Model file for the job. Use its own axes, mm. A direction names the side the tool comes from. Give positions to 0.01 mm unless a question says otherwise; leave off trailing zeros. Write each loop counter-clockwise with the first axis right and the second up, starting at its lowest first coordinate (ties: lowest second). Pieces come first, ordered by that corner, then holes. Notation, with made-up numbers: (64.25, -23.5) - (121.25, -23.5) arc R24 cw to (121.25, -12.5) - close; hole circle Ø10 at (-10, 87). An arc over 180 degrees is marked (long way). Use CSV: the item, a comma, the result in double quotes.
from build123d import *

# Parameters (mm, degrees)
SKETCH1_W           = 55
SKETCH1_H           = 46
SKETCH1_W_2         = 40
SKETCH1_H_2         = 30
BOSS_EXTRUDE1_DEPTH = 6
SKETCH3_R           = 3.556
CUT_EXTRUDE1_DEPTH  = 24
SKETCH6_W           = 12
SKETCH6_H           = 12
CUT_EXTRUDE4_DEPTH  = 4
FILLET1_R           = 10


with BuildPart() as part:
    # Sketch1 → Boss-Extrude1 (new body, symmetric)
    with BuildSketch(Plane.XY):
        Rectangle(SKETCH1_W, SKETCH1_H)
        Rectangle(SKETCH1_W_2, SKETCH1_H_2, mode=Mode.SUBTRACT)
    extrude(amount=BOSS_EXTRUDE1_DEPTH, both=True)

    # Sketch3 → Cut-Extrude1 (cut, through all)
    with BuildSketch(Plane(origin=(0, 0, 0), x_dir=(1, 0, 0), z_dir=(0, 1, 0))):
        with Locations((-8, 0)):
            Circle(SKETCH3_R)
    extrude(amount=CUT_EXTRUDE1_DEPTH, mode=Mode.SUBTRACT)

    # Sketch6 → Cut-Extrude4 (cut)
    with BuildSketch(Plane.XZ.offset(23)):
        Rectangle(SKETCH6_W, SKETCH6_H)
    extrude(amount=-CUT_EXTRUDE4_DEPTH, mode=Mode.SUBTRACT)

    # Fillet1
    fillet1_edges = [part.edges().sort_by_distance(p)[0] for p in [
        (-27.5, -23, 0),
        (-27.5, 23, 0),
        (27.5, 23, 0),
        (27.5, -23, 0),
    ]]
    fillet(fillet1_edges, radius=FILLET1_R)


solid = part.part
(1) Saw through at A-A, the plane x = -8. List the corners of the cut face in (y, z).
Checked values:
outline,"(-23, -6) - (-15, -6) - (-15, 6) - (-23, 6) - close; (15, -6) - (23, -6) - (23, -3.56) - (15, -3.56) - close; (15, 3.56) - (23, 3.56) - (23, 6) - (15, 6) - close"
(2) Saw through at D-D, the plane z = -2. List the corners of the cut face in (x, y).
Checked values:
outline,"(-27.5, -13) arc R10 ccw to (-17.5, -23) - (-6, -23) - (-6, -19) - (6, -19) - (6, -23) - (17.5, -23) arc R10 ccw to (27.5, -13) - (27.5, 13) arc R10 ccw to (17.5, 23) - (-5.06, 23) - (-5.06, 15) - (20, 15) - (20, -15) - (-20, -15) - (-20, 15) - (-10.94, 15) - (-10.94, 23) - (-17.5, 23) arc R10 ccw to (-27.5, 13) - close"
(3) 3-axis set-ups, long thin cutter, end or side, ignore diameter. For faces 4 (the face through (0, -15, 0)), 5 (the face through (27.5, 0, 0)), 6 (the face through (6, -21, 0)): which of +Z, -Z, +X, -X, +Y, -Y reach the whole face in a straight line?
Checked values:
face 4,"+Z, -Z"
face 5,"+Z, -Z, +X, +Y, -Y"
face 6,"+Z, -Z, -Y"
(4) Flat gauge pins, fed straight in: P1, Ø2, axis at y = -20, z = -2.5, coming from the -X side; P2, Ø6, axis at x = -8, z = -1, coming from the +Y side; P3, Ø2, axis at y = -21, z = -0.5, coming from the +X side; P4, Ø6, axis at x = -2.5, z = -2, coming from the -Y side. Where does each tip first touch, or does it go through?
Checked values:
P1,"stops at x = -25.5"
P2,"stops at y = 23"
P3,"stops at x = 24.64"
P4,"stops at y = -19"
(5) Pull direction Y, two halves, no side cores. Call faces 1 (the face through (-20, 0, 0)), 2 (the face through (-4.715, 18.944, 1.362)), 3 (the face through (24.49, 20.15, -0.08)): released by +Y, released by -Y, zero draft, split by the parting line, or undercut.
Checked values:
face 1,"undercut"
face 2,"zero draft"
face 3,"released by +Y"
(6) Wall check: probe 1 along Y at (x, z) = (18, -1.25); probe 2 along X at (y, z) = (7, -5.5); probe 3 along Z at (x, y) = (-8, 18). Give the ranges that are in metal, low to high. Write a range as [from, to].
Checked values:
probe 1,"y = [-22.99, -15], [15, 22.99]"
probe 2,"x = [-27.5, -20], [20, 27.5]"
probe 3,"z = [-6, -3.56], [3.56, 6]"
(7) Saw through at C-C, the plane x = 15. List the corners of the cut face in (y, z), then the cut area to 3 significant figures.
Checked values:
outline,"(-23, -6) - (-15, -6) - (-15, 6) - (-23, 6) - close; (15, -6) - (23, -6) - (23, 6) - (15, 6) - close"
area,"192 mm^2"
(8) Saw through at B-B, the plane y = -11. List the corners of the cut face in (x, z), then the cut area to 3 significant figures.
Checked values:
outline,"(-27.5, -6) - (-20, -6) - (-20, 6) - (-27.5, 6) - close; (20, -6) - (27.5, -6) - (27.5, 6) - (20, 6) - close"
area,"180 mm^2"
